CAD build for the part. Positions are in the model's coordinates, mm. A direction names the side the tool comes from. Coordinates: 2 decimals unless noted, no trailing zeros. Order: outer loops, then holes, each group sorted by start corner. A loop starts at its lowest first (then second) coordinate and runs counter-clockwise, first axis right, second up. Notation, with made-up numbers: M 37,70 L 75,70 A16 ccw 75,76 Z; hole C 65,8 d7. An arc over 180 degrees is marked long. One line per item, written item: value.
from build123d import *

# Parameters (mm, degrees)
F0_R     = 8
F0_R_2   = 2.5
F1_DEPTH = 2.5
F2_R     = 6.5
F2_R_2   = 4
F3_DEPTH = 0.5
F4_SIZE  = 0.25
F5_SIZE  = 0.1


# Not quite as in the source:
# - a pattern or mirror of a feature is missing from the dataset's text; its kind, count and spacing are read off the source's solid


with BuildPart() as f1:
    # F0 (on Front) → F1 (new body, symmetric)
    with BuildSketch(Plane.XZ):
        Circle(F0_R)
        Circle(F0_R_2, mode=Mode.SUBTRACT)
    extrude(amount=F1_DEPTH, both=True)

    # F2 (on face) → F3 (cut)
    with BuildSketch(Plane.XZ.offset(2.5)):
        Circle(F2_R)
        Circle(F2_R_2, mode=Mode.SUBTRACT)
    f3 = extrude(amount=-F3_DEPTH, mode=Mode.SUBTRACT)

    # F3_copies: F3 across plane
    add(f3.mirror(Plane.ZX), mode=Mode.SUBTRACT)

    # F4
    f4_edges = [f1.edges().sort_by_distance(p)[0] for p in [
        (-8, -2.5, 0),
        (-8, 2.5, 0),
    ]]
    chamfer(f4_edges, length=F4_SIZE)

    # F5
    f5_edges = [f1.edges().sort_by_distance(p)[0] for p in [
        (-6.5, -2.5, 0),
        (-4, -2.5, 0),
        (-6.5, 2.5, 0),
        (-4, 2.5, 0),
    ]]
    chamfer(f5_edges, length=F5_SIZE)


solid = f1.part
Q1. Mould opens along X. For faces 1 (the face through (-1.73, -0.03, -7.81)), 2 (the face through (-5.158, 2.203, -3.955)), 3 (the face through (0, -2.5, -3)) say: released by +X, released by -X, zero draft, split by the parting line, or undercut.
Recorded:
face 1: split by the parting line
face 2: undercut
face 3: zero draft
Q2. Slice it at A-A (y = 0.75). List the corners of the cut face in (x, z), plus the area to 3 significant figures.
Recorded:
outline: C 0,0 d16; hole C 0,0 d5
area: 181 mm^2
Q3. Which spindle directions (+Z, -Z, +X, -X, +Y, -Y) get a long thin tool onto all of the face, cutting with end or side? Do faces 4 (the face through (-3.5, -2.5, 5.8)), 5 (the face through (3, 2, 3)), 6 (the face through (3, -2, 3)). Say none if no direction does.
Recorded:
face 4: +Z, -Z, +X, -X, -Y
face 5: +Y
face 6: -Y
Q4. Pin check, flat tips, straight feed: pin 1 Ø1.5 at (y, z) = (-0.5, 3.5) entering from -X; pin 2 Ø3 at (x, z) = (0, 0) entering from -Y; pin 3 Ø1.5 at (y, z) = (-1, -1) entering from -X. Stop position of each tip, or through.
Recorded:
pin 1: stops at x = -7.51
pin 2: passes through
pin 3: stops at x = -8
Q5. Drill centre lines: line 1 along Z through (x, y) = (0, 2.1); line 2 along Z through (x, y) = (0, -0.65); line 3 along Z through (x, y) = (1.5, -2.15). Where is each one in solid material? Low to high.
Recorded:
line 1: z = -8 to -6.5, -4 to -2.5, 2.5 to 4, 6.5 to 8
line 2: z = -8 to -2.5, 2.5 to 8
line 3: z = -7.86 to -6.32, -3.71 to -2, 2 to 3.71, 6.32 to 7.86
